Build history of the part. All positions in model axes, mm. A direction names the side the tool comes from. Coordinates: 2 decimals unless noted, no trailing zeros. Order: outer loops, then holes, each group sorted by start corner. A loop starts at its lowest first (then second) coordinate and runs counter-clockwise, first axis right, second up. Notation, with made-up numbers: (33, -6.5) - (66, -6.5) arc R29 cw to (66, 15.5) - close; hole circle Ø2 at (36.5, -35.75). An arc over 180 degrees is marked (long way). One line per item, written item: value.
from build123d import *

# Parameters (mm, degrees)
SKETCH_1_W             = 44
SKETCH_1_H             = 29
EXTRUDE_1_DEPTH        = 23
SHELL_1_T              = -2
CUT_EXTRUDE_1_REACH    = 53.723
SKETCH_2_W             = 12
SKETCH_2_H             = 7
CUT_EXTRUDE_2_REACH    = 52.032
SKETCH_3_W             = 10
SKETCH_3_H             = 4
FILLET_1_R             = 1
FILLET_2_R             = 2
CUT_EXTRUDE_START      = -2
SKETCH_4_W             = 25
SKETCH_4_H             = 3
CUT_EXTRUDE_3_DEPTH    = 2
SKETCH_5_W             = 26.6
SKETCH_5_H             = 1.8
CUT_EXTRUDE_4_DEPTH    = 42.8
CUT_EXTRUDE_5_REACH    = 53.723
SKETCH_6_R             = 0.8
CUT_EXTRUDE_6_REACH    = 36.975
SKETCH_8_W             = 14
SKETCH_8_H             = 2
CUT_EXTRUDE_7_REACH    = 45.058
SKETCH_9_W             = 14
SKETCH_9_H             = 2
FILLET_3_R             = 1
FILLET_4_R             = 1
FILLET_3_OF_MIRROR_1_R = 1
FILLET_4_OF_MIRROR_1_R = 1


# Some blends are built 0.0001 mm under size
with BuildPart() as part:
    # 草图1 → 凸台-拉伸1 (new body)
    with BuildSketch(Plane(origin=(0, 0, 0), x_dir=(1, 0, 0), z_dir=(0, 1, 0))):
        Rectangle(SKETCH_1_W, SKETCH_1_H)
    extrude(amount=EXTRUDE_1_DEPTH)

    # 抽壳1
    shell_1_openings = [part.faces().sort_by_distance(p)[0] for p in [
        (0, 23, 0),
    ]]
    offset(amount=SHELL_1_T, openings=shell_1_openings, kind=Kind.INTERSECTION)

    # 草图2 → 切除-拉伸1 (cut, up to next)
    with BuildSketch(Plane(origin=(22, 0, 0), x_dir=(0, 0, -1), z_dir=(1, 0, 0)), mode=Mode.PRIVATE) as cut_extrude_1_sk1:
        with Locations((0, 19.5)):
            Rectangle(SKETCH_2_W, SKETCH_2_H)
    cut_extrude_1_tool1 = extrude(cut_extrude_1_sk1.sketch, amount=-CUT_EXTRUDE_1_REACH, mode=Mode.PRIVATE) & part.part
    add(cut_extrude_1_tool1.solids().sort_by_distance((22, 19.5, 0))[0], mode=Mode.SUBTRACT)

    # 草图3 → 切除-拉伸2 (cut, up to next)
    with BuildSketch(Plane(origin=(-20, 0, 0), x_dir=(0, 0, -1), z_dir=(1, 0, 0)), mode=Mode.PRIVATE) as cut_extrude_2_sk1:
        with Locations((0, 13)):
            Rectangle(SKETCH_3_W, SKETCH_3_H)
    cut_extrude_2_tool1 = extrude(cut_extrude_2_sk1.sketch, amount=-CUT_EXTRUDE_2_REACH, mode=Mode.PRIVATE) & part.part
    add(cut_extrude_2_tool1.solids().sort_by_distance((-20, 13, 0))[0], mode=Mode.SUBTRACT)

    # 圆角1
    fillet_1_edges = [part.edges().sort_by_distance(p)[0] for p in [
        (-21, 11, 5),
        (-21, 15, 5),
        (-21, 15, -5),
        (-21, 11, -5),
    ]]
    fillet(fillet_1_edges, radius=FILLET_1_R)

    # 圆角2
    fillet_2_edges = [part.edges().sort_by_distance(p)[0] for p in [
        (21, 16, 6),
        (21, 16, -6),
    ]]
    fillet(fillet_2_edges, radius=FILLET_2_R)

    # 草图4 → 切除-拉伸3 (cut)
    with BuildSketch(Plane(origin=(22, 0, 0), x_dir=(0, 0, -1), z_dir=(1, 0, 0)).offset(CUT_EXTRUDE_START)):
        with Locations((0, 21.5)):
            Rectangle(SKETCH_4_W, SKETCH_4_H)
    extrude(amount=CUT_EXTRUDE_3_DEPTH, mode=Mode.SUBTRACT)

    # 草图5 → 切除-拉伸4 (cut)
    with BuildSketch(Plane(origin=(22, 0, 0), x_dir=(0, 0, -1), z_dir=(1, 0, 0))):
        with Locations((0, 20.9)):
            Rectangle(SKETCH_5_W, SKETCH_5_H)
    extrude(amount=-CUT_EXTRUDE_4_DEPTH, mode=Mode.SUBTRACT)

    # 草图6 → 切除-拉伸5 (cut, up to next)
    with BuildSketch(Plane.ZY.offset(22), mode=Mode.PRIVATE) as cut_extrude_5_sk1:
        with Locations((-8.5, 20.9)):
            Circle(SKETCH_6_R)
    cut_extrude_5_tool1 = extrude(cut_extrude_5_sk1.sketch, amount=-CUT_EXTRUDE_5_REACH, mode=Mode.PRIVATE) & part.part
    # 草图6 → 切除-拉伸5 (cut, up to next)
    with BuildSketch(Plane.ZY.offset(22), mode=Mode.PRIVATE) as cut_extrude_5_sk2:
        with Locations((8.5, 20.9)):
            Circle(SKETCH_6_R)
    cut_extrude_5_tool2 = extrude(cut_extrude_5_sk2.sketch, amount=-CUT_EXTRUDE_5_REACH, mode=Mode.PRIVATE) & part.part
    add(cut_extrude_5_tool1.solids().sort_by_distance((-22, 20.9, -8.5))[0], mode=Mode.SUBTRACT)
    add(cut_extrude_5_tool2.solids().sort_by_distance((-22, 20.9, 8.5))[0], mode=Mode.SUBTRACT)

    # 草图8 → 切除-拉伸6 (cut, up to next)
    with BuildSketch(Plane.XZ, mode=Mode.PRIVATE) as cut_extrude_6_sk1:
        with Locations((0, -11.5)):
            Rectangle(SKETCH_8_W, SKETCH_8_H)
    cut_extrude_6_tool1 = extrude(cut_extrude_6_sk1.sketch, amount=-CUT_EXTRUDE_6_REACH, mode=Mode.PRIVATE) & part.part
    cut_extrude_6 = cut_extrude_6_tool1.solids().sort_by_distance((0, 0, -11.5))[0]
    add(cut_extrude_6, mode=Mode.SUBTRACT)

    # 草图9 → 切除-拉伸7 (cut, up to next)
    with BuildSketch(Plane(origin=(0, 0, -14.5), x_dir=(-1, 0, 0), z_dir=(0, 0, -1)), mode=Mode.PRIVATE) as cut_extrude_7_sk1:
        with Locations((0, 3)):
            Rectangle(SKETCH_9_W, SKETCH_9_H)
    cut_extrude_7_tool1 = extrude(cut_extrude_7_sk1.sketch, amount=-CUT_EXTRUDE_7_REACH, mode=Mode.PRIVATE) & part.part
    cut_extrude_7 = cut_extrude_7_tool1.solids().sort_by_distance((0, 3, -14.5))[0]
    add(cut_extrude_7, mode=Mode.SUBTRACT)

    # 圆角3
    # the kernel refuses this fillet: 1 mm, written as the material it adds along each edge
    with BuildSketch(Plane(origin=(-7, 4, -14.5), x_dir=(0, -1, 0), z_dir=(0, 0, 1)), Plane(origin=(-7, 2, -14.5), x_dir=(1, 0, 0), z_dir=(0, 0, 1)), Plane(origin=(7, 2, -14.5), x_dir=(0, 1, 0), z_dir=(0, 0, 1))) as fillet_3_piece_1:
        with BuildLine():
            CenterArc((FILLET_3_R, FILLET_3_R), FILLET_3_R, 180, 90)
            Line((0, FILLET_3_R), (0, 0))
            Line((0, 0), (FILLET_3_R, 0))
        make_face()
    extrude(amount=2)
    with BuildSketch(Plane(origin=(7, 4, -14.5), x_dir=(0, -1, 0), z_dir=(0, 0, 1))) as fillet_3_piece_2:
        with BuildLine():
            CenterArc((FILLET_3_R, -FILLET_3_R), FILLET_3_R, 90, 90)
            Line((0, -FILLET_3_R), (0, 0))
            Line((0, 0), (FILLET_3_R, 0))
        make_face()
    extrude(amount=2)

    # 圆角4
    fillet_4_edges = [part.edges().sort_by_distance(p)[0] for p in [
        (-7, 1, -12.5),
        (-7, 1, -10.5),
        (7, 1, -12.5),
        (7, 1, -10.5),
    ]]
    fillet(fillet_4_edges, radius=FILLET_4_R - 0.0001)  # a hair under: the kernel refuses the full size

    # 镜向1: 切除-拉伸6, 切除-拉伸7 across plane
    add(cut_extrude_6.mirror(Plane.XY), mode=Mode.SUBTRACT)
    add(cut_extrude_7.mirror(Plane.XY), mode=Mode.SUBTRACT)

    # 圆角3 of 镜向1
    # the kernel refuses this fillet: 1 mm, written as the material it adds along each edge
    with BuildSketch(Plane(origin=(-7, 4, 14.5), x_dir=(1, 0, 0), z_dir=(0, 0, -1)), Plane(origin=(-7, 2, 14.5), x_dir=(0, 1, 0), z_dir=(0, 0, -1)), Plane(origin=(7, 2, 14.5), x_dir=(-1, 0, 0), z_dir=(0, 0, -1))) as fillet_3_of_mirror_1_piece_1:
        with BuildLine():
            CenterArc((FILLET_3_OF_MIRROR_1_R, FILLET_3_OF_MIRROR_1_R), FILLET_3_OF_MIRROR_1_R, 180, 90)
            Line((0, FILLET_3_OF_MIRROR_1_R), (0, 0))
            Line((0, 0), (FILLET_3_OF_MIRROR_1_R, 0))
        make_face()
    extrude(amount=2)
    with BuildSketch(Plane(origin=(7, 4, 14.5), x_dir=(-1, 0, 0), z_dir=(0, 0, -1))) as fillet_3_of_mirror_1_piece_2:
        with BuildLine():
            CenterArc((FILLET_3_OF_MIRROR_1_R, -FILLET_3_OF_MIRROR_1_R), FILLET_3_OF_MIRROR_1_R, 90, 90)
            Line((0, -FILLET_3_OF_MIRROR_1_R), (0, 0))
            Line((0, 0), (FILLET_3_OF_MIRROR_1_R, 0))
        make_face()
    extrude(amount=2)

    # 圆角4 of 镜向1
    fillet_4_of_mirror_1_edges = [part.edges().sort_by_distance(p)[0] for p in [
        (-7, 1, 12.5),
        (-7, 1, 10.5),
        (7, 1, 12.5),
        (7, 1, 10.5),
    ]]
    fillet(fillet_4_of_mirror_1_edges, radius=FILLET_4_OF_MIRROR_1_R - 0.0001)  # a hair under: the kernel refuses the full size


solid = part.part
1. Band-saw the part on C-C, the plane y = 3. Give the cut face in (x, z).
Values found:
outline: (-22, -14.5) - (-7, -14.5) - (-7, -12.5) - (-20, -12.5) - (-20, 12.5) - (-7, 12.5) - (-7, 14.5) - (-22, 14.5) - close; (7, -14.5) - (22, -14.5) - (22, 14.5) - (7, 14.5) - (7, 12.5) - (20, 12.5) - (20, -12.5) - (7, -12.5) - close
2. Band-saw the part on D-D, the plane x = -8. Give the cut face in (y, z).
Values found:
outline: (0, -14.5) - (23, -14.5) - (23, -12.5) - (21.8, -12.5) - (21.8, -13.3) - (20, -13.3) - (20, -12.5) - (2, -12.5) - (2, 12.5) - (20, 12.5) - (20, 13.3) - (21.8, 13.3) - (21.8, 12.5) - (23, 12.5) - (23, 14.5) - (0, 14.5) - close
3. Two-plate mould, pull along X, no slides. Class faces 1 (the face through (-22, 9, 0)), 2 (the face through (-3, 23, 13)), 3 (the face through (6.699, 1.014, -12.215)): pulls with the +X half, pulls with the -X half, needs draft (parallel to the pull), parting line crosses it, or undercut.
Values found:
face 1: pulls with the -X half
face 2: needs draft
face 3: undercut
4. Band-saw the part on A-A, the plane y = 20.9. Give the cut face in (x, z), and give its area (3 significant figures).
Values found:
outline: (-22, -14.5) - (22, -14.5) - (22, -13.3) - (-20.8, -13.3) - (-20.8, -9.3) - (-22, -9.3) - close; (-22, -7.7) - (-20.8, -7.7) - (-20.8, 7.7) - (-22, 7.7) - close; (-22, 9.3) - (-20.8, 9.3) - (-20.8, 13.3) - (22, 13.3) - (22, 14.5) - (-22, 14.5) - close
area: 134 mm2
5. Flat gauge pins, fed straight in: P1, Ø1, axis at x = -12.5, z = -10, coming from the +Y side; P2, Ø0.5, axis at y = 21, z = 6.5, coming from the +X side. Where does each tip first touch, or does it go through?
Values found:
P1: stops at y = 2
P2: stops at x = -20.8
6. 3-axis set-ups, long thin cutter, end or side, ignore diameter. For faces 4 (the face through (0, 10, 12.5)), 5 (the face through (20.99, 16.6, -5.43)), 6 (the face through (-6.715, 1.014, -10.801)), 7 (the face through (-21, 13, -5)), 8 (the face through (0, 2, 14)): which of +Z, -Z, +X, -X, +Y, -Y reach the whole face in a straight line?
Values found:
face 4: +Y
face 5: +X, +Y
face 6: +Y, -Y
face 7: -X
face 8: +Z, -Z
7. Probe line 1 along X through (y, z) = (3.5, -6.75); line 2 along Y through (x, z) = (-21.35, -8.5); line 3 along X through (y, z) = (20.25, 10.75). List the from-to ranges inside material, lowest first.
Values found:
line 1: x = -22 to -20, 20 to 22
line 2: y = 0 to 20.1, 21.7 to 23
line 3: x = -22 to -20.8
8. Band-saw the part on B-B, the plane z = -8.5. Give the cut face in (x, y), and give its area (3 significant figures).
Values found:
outline: (-22, 0) - (22, 0) - (22, 20) - (20, 20) - (20, 2) - (-20, 2) - (-20, 20) - (-20.8, 20) - (-20.8, 20.1) - (-22, 20.1) - close; (-22, 21.7) - (-20.8, 21.7) - (-20.8, 21.8) - (-20, 21.8) - (-20, 23) - (-22, 23) - close
area: 163 mm2
